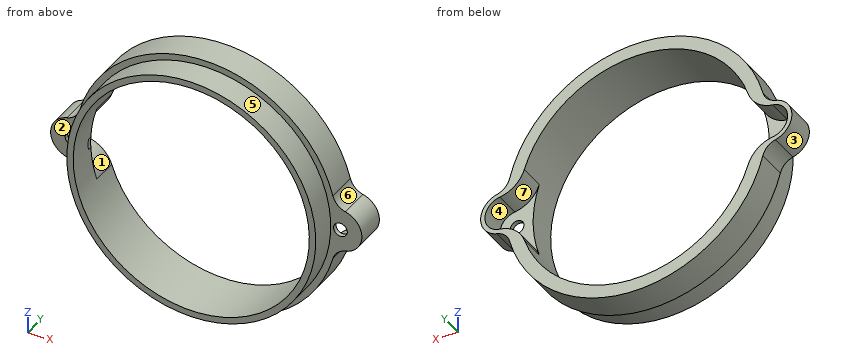
```python
from build123d import *

# Parameters (mm, degrees)
SKETCH1_R           = 29
SKETCH1_R_2         = 27.5
BOSS_EXTRUDE1_DEPTH = 6
SKETCH3_R           = 30.5
SKETCH3_R_2         = 27.5
BOSS_EXTRUDE3_DEPTH = 7
BOSS_EXTRUDE4_START = -6
BOSS_EXTRUDE4_DEPTH = 6
CUT_EXTRUDE1_START  = -7
SKETCH6_R           = 4
CUT_EXTRUDE1_DEPTH  = 7
BOSS_EXTRUDE5_START = 1
SKETCH8_R           = 4
SKETCH8_R_2         = 1.6
BOSS_EXTRUDE5_DEPTH = 1
CUT_EXTRUDE2_START  = -6
CUT_EXTRUDE2_DEPTH  = 6
CUT_EXTRUDE3_START  = -10
SKETCH10_R          = 27.5
CUT_EXTRUDE3_DEPTH  = 10
CIRPATTERN1_COUNT   = 2


with BuildPart() as part:
    # Sketch1 → Boss-Extrude1 (new body)
    with BuildSketch(Plane(origin=(0, 0, 0), x_dir=(1, 0, 0), z_dir=(0, 1, 0))):
        with Locations(Location((0, 0, 0), (0, 0, 270))):
            Circle(SKETCH1_R)
        with Locations(Location((0, 0, 0), (0, 0, 270))):
            Circle(SKETCH1_R_2, mode=Mode.SUBTRACT)
    extrude(amount=BOSS_EXTRUDE1_DEPTH)

    # Sketch3 → Boss-Extrude3 (add)
    with BuildSketch(Plane(origin=(0, 6, 0), x_dir=(1, 0, 0), z_dir=(0, 1, 0))):
        with Locations(Location((0, 0, 0), (0, 0, 270))):
            Circle(SKETCH3_R)
        with Locations(Location((0, 0, 0), (0, 0, 270))):
            Circle(SKETCH3_R_2, mode=Mode.SUBTRACT)
    extrude(amount=BOSS_EXTRUDE3_DEPTH)

    # Sketch4 → Boss-Extrude4 (add)
    with BuildSketch(Plane(origin=(0, 13, 0), x_dir=(1, 0, 0), z_dir=(0, 1, 0)).offset(BOSS_EXTRUDE4_START)):
        with BuildLine():
            ThreePointArc((-30.253, -3.873756704), (-35.25, 0), (-30.253, 3.873756704))
            ThreePointArc((-30.253, 3.873756704), (-30.245409649, 3.932581236), (-30.237704918, 3.991390897))
            ThreePointArc((-30.237704918, 3.991390897), (-29.929181214, 5.873168807), (-29.503666667, 7.731988956))
            ThreePointArc((-29.503666667, 7.731988956), (-30.570387885, 5.892011652), (-32.429444444, 4.858900164))
            ThreePointArc((-32.429444444, 4.858900164), (-36.25, 0), (-32.429444444, -4.858900164))
            ThreePointArc((-32.429444444, -4.858900164), (-30.570387885, -5.892011652), (-29.503666667, -7.731988956))
            ThreePointArc((-29.503666667, -7.731988956), (-29.929181214, -5.873168807), (-30.237704918, -3.991390897))
            ThreePointArc((-30.237704918, -3.991390897), (-30.245409649, -3.932581236), (-30.253, -3.873756704))
        make_face()
    boss_extrude4 = extrude(amount=BOSS_EXTRUDE4_DEPTH)

    # Sketch6 → Cut-Extrude1 (cut)
    with BuildSketch(Plane(origin=(0, 13, 0), x_dir=(1, 0, 0), z_dir=(0, 1, 0)).offset(CUT_EXTRUDE1_START)):
        with Locations((-31.25, 0)):
            Circle(SKETCH6_R)
    cut_extrude1 = extrude(amount=CUT_EXTRUDE1_DEPTH, mode=Mode.SUBTRACT)

    # Sketch8 → Boss-Extrude5 (add)
    # profile 1 of 2: a face of its own
    with BuildSketch(Plane.XZ.offset(-7).offset(BOSS_EXTRUDE5_START)):
        with Locations((-31.25, 0)):
            Circle(SKETCH8_R)
        with Locations(Location((-31.25, 0, 0), (0, 0, 270))):
            Circle(SKETCH8_R_2, mode=Mode.SUBTRACT)
    # profile 2 of 2: a face of its own
    with BuildSketch(Plane.XZ.offset(-7).offset(BOSS_EXTRUDE5_START)):
        with BuildLine():
            ThreePointArc((-30.253, -3.873756704), (-29.94054595, -5.814955562), (-29.503666667, -7.731988956))
            ThreePointArc((-29.503666667, -7.731988956), (-30.570387885, -5.892011652), (-32.429444444, -4.858900164))
            ThreePointArc((-32.429444444, -4.858900164), (-36.25, 0), (-32.429444444, 4.858900164))
            ThreePointArc((-32.429444444, 4.858900164), (-30.570387885, 5.892011652), (-29.503666667, 7.731988956))
            ThreePointArc((-29.503666667, 7.731988956), (-29.94054595, 5.814955562), (-30.253, 3.873756704))
            ThreePointArc((-30.253, 3.873756704), (-35.25, 0), (-30.253, -3.873756704))
        make_face()
    boss_extrude5 = extrude(amount=-BOSS_EXTRUDE5_DEPTH)

    # Sketch9 → Cut-Extrude2 (cut)
    with BuildSketch(Plane(origin=(0, 13, 0), x_dir=(1, 0, 0), z_dir=(0, 1, 0)).offset(CUT_EXTRUDE2_START)):
        with BuildLine():
            ThreePointArc((-27.469, 1.305388448), (-27.033467309, 5.04397118), (-26.091521739, 8.688066145))
            ThreePointArc((-26.091521739, 8.688066145), (-28.264861577, 5.511091819), (-31.789272727, 3.963481415))
            ThreePointArc((-31.789272727, 3.963481415), (-29.15391711, 3.406822055), (-27.469, 1.305388448))
        make_face()
        with BuildLine():
            ThreePointArc((-31.789272727, -3.963481415), (-28.264861577, -5.511091819), (-26.091521739, -8.688066145))
            ThreePointArc((-26.091521739, -8.688066145), (-27.033467309, -5.04397118), (-27.469, -1.305388448))
            ThreePointArc((-27.469, -1.305388448), (-29.15391711, -3.406822055), (-31.789272727, -3.963481415))
        make_face()
    cut_extrude2 = extrude(amount=CUT_EXTRUDE2_DEPTH, mode=Mode.SUBTRACT)

    # Sketch10 → Cut-Extrude3 (cut)
    with BuildSketch(Plane(origin=(0, 7, 0), x_dir=(1, 0, 0), z_dir=(0, 1, 0)).offset(CUT_EXTRUDE3_START)):
        with Locations(Location((0, 0, 0), (0, 0, 161.583053277))):
            Circle(SKETCH10_R)
    cut_extrude3 = extrude(amount=CUT_EXTRUDE3_DEPTH, mode=Mode.SUBTRACT)

    # CirPattern1: Boss-Extrude4, Cut-Extrude1, Boss-Extrude5, Cut-Extrude2, Cut-Extrude3 ×2 about axis
    cirpattern1_axis = Axis((0, 0, 0), (0, 1, 0))
    add([boss_extrude4.rotate(cirpattern1_axis, i * 360 / CIRPATTERN1_COUNT) for i in range(1, CIRPATTERN1_COUNT)])
    add([cut_extrude1.rotate(cirpattern1_axis, i * 360 / CIRPATTERN1_COUNT) for i in range(1, CIRPATTERN1_COUNT)], mode=Mode.SUBTRACT)
    add([boss_extrude5.rotate(cirpattern1_axis, i * 360 / CIRPATTERN1_COUNT) for i in range(1, CIRPATTERN1_COUNT)])
    add([cut_extrude2.rotate(cirpattern1_axis, i * 360 / CIRPATTERN1_COUNT) for i in range(1, CIRPATTERN1_COUNT)], mode=Mode.SUBTRACT)
    add([cut_extrude3.rotate(cirpattern1_axis, i * 360 / CIRPATTERN1_COUNT) for i in range(1, CIRPATTERN1_COUNT)], mode=Mode.SUBTRACT)


solid = part.part
```
Verification items for the finished model (mm, model axes). Face numbers are marked on the shaded views. A direction names the side the tool comes from. Round coordinates to 2 decimals unless told otherwise and drop trailing zeros. Order: outer loops, then holes, each group sorted by start corner. A loop starts at its lowest first (then second) coordinate and runs counter-clockwise, first axis right, second up. Notation, with made-up numbers: (-39.75, -7) - (12.25, -7) arc R16 ccw to (12.25, 24) - close; hole circle Ø1 at (43, 19). An arc over 180 degrees is marked (long way). Use CSV: the item, a comma, the result in double quotes.
(1) Section check D-D on y = 3. Record the boundary of the cut face in (x, z), and give its area (3 significant figures).
Entries:
outline,"circle Ø58 at (0, 0); hole circle Ø55 at (0, 0)"
area,"266 mm^2"
(2) Gauge pin test, flat ends, axial feed: pin 1 Ø3 at (x, y) = (28.5, 10.5) entering from -Z; pin 2 Ø5 at (y, z) = (2, 23) entering from -X; pin 3 Ø4.5 at (x, z) = (-31.5, 2) entering from +Y; pin 4 Ø5 at (y, z) = (10, 4) entering from +X. Record the tip position at first contact, or that the pin passes through.
Entries:
pin 1,"z = -14.19"
pin 2,"x = -20.51"
pin 3,"y = 13"
pin 4,"x = 36.02"
(3) Section check C-C on z = 10. Record the boundary of the cut face in (x, y), and give its area (3 significant figures).
Entries:
outline,"(-28.81, 6) - (-27.22, 6) - (-27.22, 0) - (-25.62, 0) - (-25.62, 13) - (-28.81, 13) - close; (25.62, 0) - (27.22, 0) - (27.22, 6) - (28.81, 6) - (28.81, 13) - (25.62, 13) - close"
area,"64.0 mm^2"
(4) Section check B-B on x = 8. Record the boundary of the cut face in (y, z), and give its area (3 significant figures).
Entries:
outline,"(0, -27.87) - (6, -27.87) - (6, -29.43) - (13, -29.43) - (13, -26.31) - (0, -26.31) - close; (0, 26.31) - (13, 26.31) - (13, 29.43) - (6, 29.43) - (6, 27.87) - (0, 27.87) - close"
area,"62.5 mm^2"
(5) Mould release check, pull along Z, two halves, no side actions. Record for the marked faces 4, 5, 6 and 7: released by +Z, released by -Z, zero draft, split by the parting line, or undercut.
Entries:
face 4,"undercut"
face 5,"split by the parting line"
face 6,"released by +Z"
face 7,"undercut"
(6) Access from +Z, -Z, +X, -X, +Y, -Y to the whole of each face (thin tool, end or side, straight path). Record for the marked faces 1, 2 and 3.
Entries:
face 1,"+Y"
face 2,"-Y"
face 3,"-X, +Y, -Y"
(7) Thickness scan on probe 1 along X at (y, z) = (6.3, 0); probe 2 along Z at (x, y) = (0, 9.5); probe 3 along Z at (x, y) = (31.25, 6.85). Record the ranges inside material, lowest first. Write a range as from..to.
Entries:
probe 1,"-36.25..-32.85, -29.65..-27.5, 27.5..29.65, 32.85..36.25"
probe 2,"-30.5..-27.5, 27.5..30.5"
probe 3,"-5.36..-1.6, 1.6..5.36"
(8) Section check A-A on y = 8. Record the boundary of the cut face in (x, z).
Entries:
outline,"(-32.43, -4.86) arc R4 cw to (-29.5, -7.73) arc R30.5 ccw to (29.5, -7.73) arc R4 cw to (32.43, -4.86) arc R5 ccw to (32.43, 4.86) arc R4 cw to (29.5, 7.73) arc R30.5 ccw to (-29.5, 7.73) arc R4 cw to (-32.43, 4.86) arc R5 ccw to start; hole (-31.79, -3.96) arc R7 cw to (-26.09, -8.69) arc R27.5 ccw to (26.09, -8.69) arc R7 cw to (31.79, -3.96) arc R4 ccw to (31.79, 3.96) arc R7 cw to (26.09, 8.69) arc R27.5 ccw to (-26.09, 8.69) arc R7 cw to (-31.79, 3.96) arc R4 ccw to start"
